Verification items for the finished model (mm, model axes). A direction names the side the tool comes from. Give positions to 0.01 mm unless a question says otherwise; leave off trailing zeros. Order: outer loops, then holes, each group sorted by start corner. A loop starts at its lowest first (then second) coordinate and runs counter-clockwise, first axis right, second up. Notation, with made-up numbers: (-2.5, 47) -> (34.5, 47) arc R18 ccw to (34.5, 66) -> close; hole circle Ø4 at (-4.75, 38.5). An arc over 180 degrees is marked (long way). Write each question's results on one line, items separated by ' | '. Start each with the question number.
1. Cross-section at B-B, the plane y = 40. Enter the section's corners in (x, z), then the cut area to 3 significant figures.
2. Set-up check for faces 1 (the face through (-4.56, 74.7, 43.07)), 2 (the face through (-81, 23, 36)), 3 (the face through (80, 53, 36)), 4 (the face through (43.5, 11, 36)), 5 (the face through (-66, 53, 36)): record each of +Z, -Z, +X, -X, +Y, -Y from which the full face is reachable in a straight line by a thin tool's end or side.
3. Depth check by flat-ended pin: pin 1 Ø6 at (x, y) = (-59, 28) entering from -Z; pin 2 Ø24 at (x, z) = (-86, 17.5) entering from -Y; pin 3 Ø2 at (y, z) = (67.5, 7.5) entering from +X; pin 4 Ø4 at (x, z) = (-31.5, 10.5) entering from +Y. Enter the tip coordinate at first touch or a pass-through.
4. Material ranges on L1, parallel to X at y = 39.5, z = 39; L2, parallel to X at y = 47, z = 56.5; L3, parallel to Z at x = 87, y = 24.5, recorded low to high. Write a range as from..to.
5. Cross-section at C-C, the plane x = -86. Enter the section's corners in (y, z).
6. Mould release check, pull along Z, two halves, no side actions. Record for faces 6 (the face through (-67.121, 37.79, 42.685)), 7 (the face through (-15, 25, 13)), 8 (the face through (-1, 0, 36)): +Z half, -Z half, draft (parallel to the pull), parting line (faces both ways), or undercut.
7. Cross-section at A-A, the plane z = 56.5. Enter the section's corners in (x, y).
8. Cross-section at D-D, the plane z = 5. Enter the section's corners in (x, y), then the cut area to 3 significant figures.
from build123d import *

# Parameters (mm, degrees)
SKETCH_1_R          = 35
EXTRUDE_1_DEPTH     = 74
SKETCH_2_R          = 35
SKETCH_2_R_2        = 21
EXTRUDE_2_DEPTH     = 13
SKETCH_3_R          = 7.5
SKETCH_3_R_2        = 5
CUT_EXTRUDE_1_DEPTH = 30


with BuildPart() as part:
    # 草图1 → 凸台-拉伸1 (new body)
    with BuildSketch(Plane.XY):
        with BuildLine():
            Line((-43.5, 0), (43.5, 0))
            Line((43.5, 0), (43.5, 23))
            Line((43.5, 23), (103.5, 23))
            Line((103.5, 23), (103.5, 53))
            Line((103.5, 53), (43.081318457, 53))
            ThreePointArc((43.081318457, 53), (0, 85), (-43.081318457, 53))
            Line((-43.081318457, 53), (-103.5, 53))
            Line((-103.5, 53), (-103.5, 23))
            Line((-103.5, 23), (-43.5, 23))
            Line((-43.5, 23), (-43.5, 0))
        make_face()
        with Locations((0, 40)):
            Circle(SKETCH_1_R, mode=Mode.SUBTRACT)
    extrude(amount=EXTRUDE_1_DEPTH)

    # 草图2 → 凸台-拉伸2 (add)
    with BuildSketch(Plane(origin=(0, 0, 0), x_dir=(-1, 0, 0), z_dir=(0, 0, -1))):
        with Locations((0, 40)):
            Circle(SKETCH_2_R)
        with Locations((0, 40)):
            Circle(SKETCH_2_R_2, mode=Mode.SUBTRACT)
    extrude(amount=-EXTRUDE_2_DEPTH)

    # 草图3 → 切除-拉伸1 (cut)
    with BuildSketch(Plane.XZ.offset(-23)):
        with Locations(Location((-86, 56.5, 0), (0, 0, 270))):
            Circle(SKETCH_3_R)
        with Locations(Location((-70.5, 39, 0), (0, 0, 270))):
            Circle(SKETCH_3_R_2)
        with Locations(Location((-86, 17.5, 0), (0, 0, 270))):
            Circle(SKETCH_3_R)
        with Locations(Location((86, 56.5, 0), (0, 0, 270))):
            Circle(SKETCH_3_R)
        with Locations(Location((70.5, 39, 0), (0, 0, 270))):
            Circle(SKETCH_3_R_2)
        with Locations(Location((86, 17.5, 0), (0, 0, 270))):
            Circle(SKETCH_3_R)
    extrude(amount=-CUT_EXTRUDE_1_DEPTH, mode=Mode.SUBTRACT)


solid = part.part
Results below:
1) outline: (-103.5, 0) -> (-21, 0) -> (-21, 13) -> (-35, 13) -> (-35, 74) -> (-103.5, 74) -> close; (21, 0) -> (103.5, 0) -> (103.5, 74) -> (35, 74) -> (35, 13) -> (21, 13) -> close; hole circle Ø15 at (-86, 17.5); hole circle Ø15 at (-86, 56.5); hole circle Ø10 at (-70.5, 39); hole circle Ø10 at (70.5, 39); hole circle Ø15 at (86, 17.5); hole circle Ø15 at (86, 56.5) | area: 9,640 mm²
2) face 1: +Z | face 2: +Z, -Z, -X, -Y | face 3: +Z, -Z, +X, +Y | face 4: +Z, -Z, +X, -Y | face 5: +Z, -Z, -X, +Y
3) pin 1: stops at z = 0 | pin 2: stops at y = 23 | pin 3: stops at x = 36.37 | pin 4: stops at y = 73.98
4) L1: x = -103.5..-75.5, -65.5..-35, 35..65.5, 75.5..103.5 | L2: x = -103.5..-93.5, -78.5..-34.29, 34.29..78.5, 93.5..103.5 | L3: z = 0..10.07, 24.93..49.07, 63.93..74
5) outline: (23, 0) -> (53, 0) -> (53, 10) -> (23, 10) -> close; (23, 25) -> (53, 25) -> (53, 49) -> (23, 49) -> close; (23, 64) -> (53, 64) -> (53, 74) -> (23, 74) -> close
6) face 6: undercut | face 7: +Z half | face 8: draft
7) outline: (-103.5, 23) -> (-93.5, 23) -> (-93.5, 53) -> (-103.5, 53) -> close; (-78.5, 23) -> (-43.5, 23) -> (-43.5, 0) -> (43.5, 0) -> (43.5, 23) -> (78.5, 23) -> (78.5, 53) -> (43.08, 53) arc R45 ccw to (-43.08, 53) -> (-78.5, 53) -> close; (93.5, 23) -> (103.5, 23) -> (103.5, 53) -> (93.5, 53) -> close; hole circle Ø70 at (0, 40)
8) outline: (-103.5, 23) -> (-43.5, 23) -> (-43.5, 0) -> (43.5, 0) -> (43.5, 23) -> (103.5, 23) -> (103.5, 53) -> (43.08, 53) arc R45 ccw to (-43.08, 53) -> (-103.5, 53) -> close; hole circle Ø42 at (0, 40) | area: 8,850 mm²
